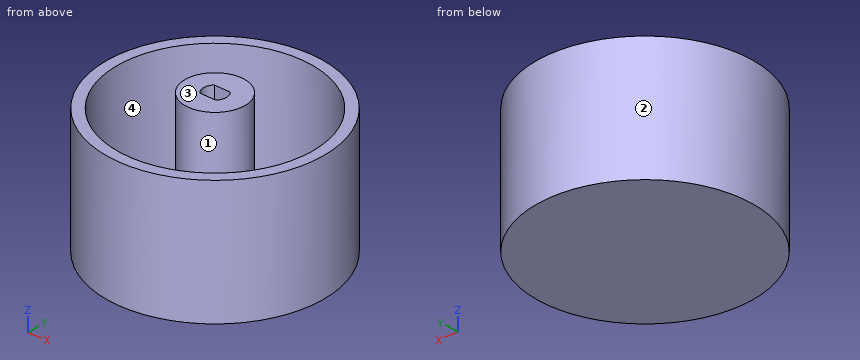
Autodesk Inventor part; units mm, degrees
ref_plane "YZ Plane" through (0, 0, 0) normal (1, 0, 0) x (0, 1, 0)
ref_plane "XZ Plane" through (0, 0, 0) normal (0, 1, 0) x (-1, 0, 0)
ref_plane "XY Plane" through (0, 0, 0) normal (0, 0, 1) x (1, 0, 0)
sketch "Sketch1" plane through (0, 0, 0) normal (0, 0, 1) x (1, 0, 0)
  circle A0 centre (0, 0) radius 25.4
  dimension "d0" = 50.8
extrude "Extrusion1" add sketch "Sketch1" along normal blind 3.81
sketch "Sketch2" plane through (0, 0, 3.81) normal (0, 0, 1) x (1, 0, 0)
  circle A0 centre (0, 0) radius 22.86
  circle A1 centre (0, 0) radius 25.4
  dimension "d3" = 45.72
extrude "Extrusion2" add sketch "Sketch2" along normal blind 25.4
sketch "Sketch3" plane through (0, 0, 3.81) normal (0, 0, 1) x (1, 0, 0)
  circle A0 centre (0, 0) radius 6.985
  dimension "d6" = 13.97
extrude "Extrusion3" add sketch "Sketch3" along normal blind 28.575
sketch "Sketch4" plane through (0, 0, 32.385) normal (0, 0, 1) x (1, 0, 0)
  line L0 (-1.8665, 1.905) -> (1.8665, 1.905)
  line L1 (1.8665, -1.905) -> (-1.8665, -1.905)
  arc A0 (-1.8665, 1.905) -> (-1.8665, -1.905) centre (0, 0) ccw
  arc A1 (1.8665, -1.905) -> (1.8665, 1.905) centre (0, 0) ccw
  point P0 (0, 1.905)
  point P1 (0, -1.905)
  dimension "d10" = 1.905
  dimension "d11" = 1.905
extrude "Extrusion4" cut sketch "Sketch4" against normal blind 25.4
properties part number "Wheel" material "ABS Plastic"
Part model, mm, in its own coordinate system. Face numbers are marked on the shaded views. Give positions to 0.01 mm unless a question says otherwise; leave off trailing zeros. Loops run counter-clockwise (first coordinate to the right, second up) from the corner with the lowest first, then second, coordinate; pieces in that order, holes last. Notation, with made-up numbers: M 53.25,81.5 L 81.25,81.5 A25 ccw 81.25,93.5 Z; hole C -29,31 d4. An arc over 180 degrees is marked long. Return JSON: item names as keys, results as strings.
1) Saw through at A-A, the plane z = 28.5. List the corners of the cut face in (x, y) (1 decimal).
Calculated:
{"outline": "C 0,0 d50.8; C 0,0 d14; hole C 0,0 d45.7; hole M -1.9,-1.9 L 1.9,-1.9 A2.7 ccw 1.9,1.9 L -1.9,1.9 A2.7 ccw Z"}
2) Pull direction X, two halves, no side cores. Call the marked faces 1, 2, 3 and 4: released by +X, released by -X, zero draft, split by the parting line, or undercut.
Calculated:
{"face 1": "undercut", "face 2": "split by the parting line", "face 3": "zero draft", "face 4": "undercut"}
3) Saw through at D-D, the plane x = 19.5. List the corners of the cut face in (y, z).
Calculated:
{"outline": "M -16.28,0 L 16.28,0 L 16.28,29.21 L 11.93,29.21 L 11.93,3.81 L -11.93,3.81 L -11.93,29.21 L -16.28,29.21 Z"}
4) Drill centre lines: line 1 (Y direction, x = 0, z = 24) (3 decimals); line 2 (X direction, y = 0.5, z = 16.5); line 3 (X direction, y = -4, z = 7). Where is each one in solid material? Low to high.
Calculated:
{"line 1": "y = -25.4 to -22.86, -6.985 to -1.905, 1.905 to 6.985, 22.86 to 25.4", "line 2": "x = -25.4 to -22.85, -6.97 to -2.62, 2.62 to 6.97, 22.85 to 25.4", "line 3": "x = -25.08 to -22.51, -5.73 to 5.73, 22.51 to 25.08"}
5) Flat gauge pins, fed straight in: pin 1 Ø1 at (x, y) = (-6.5, -12.5) entering from +Z; pin 2 Ø2 at (y, z) = (-17.5, 18.5) entering from +X; pin 3 Ø3 at (x, z) = (-0.5, 16) entering from -Y. Where does each tip first touch, or does it go through?
Calculated:
{"pin 1": "stops at z = 3.81", "pin 2": "stops at x = 19.31", "pin 3": "stops at y = -25.4"}
6) Saw through at B-B, the plane x = 0. List the corners of the cut face in (y, z) (3 decimals).
Calculated:
{"outline": "M -25.4,0 L 25.4,0 L 25.4,29.21 L 22.86,29.21 L 22.86,3.81 L 6.985,3.81 L 6.985,32.385 L 1.905,32.385 L 1.905,6.985 L -1.905,6.985 L -1.905,32.385 L -6.985,32.385 L -6.985,3.81 L -22.86,3.81 L -22.86,29.21 L -25.4,29.21 Z"}
7) Saw through at C-C, the plane y = 0. List the corners of the cut face in (x, z) (3 decimals), then the cut area to 3 significant figures.
Calculated:
{"outline": "M -25.4,0 L 25.4,0 L 25.4,29.21 L 22.86,29.21 L 22.86,3.81 L 6.985,3.81 L 6.985,32.385 L 2.667,32.385 L 2.667,6.985 L -2.667,6.985 L -2.667,32.385 L -6.985,32.385 L -6.985,3.81 L -22.86,3.81 L -22.86,29.21 L -25.4,29.21 Z", "area": "586 mm2"}
